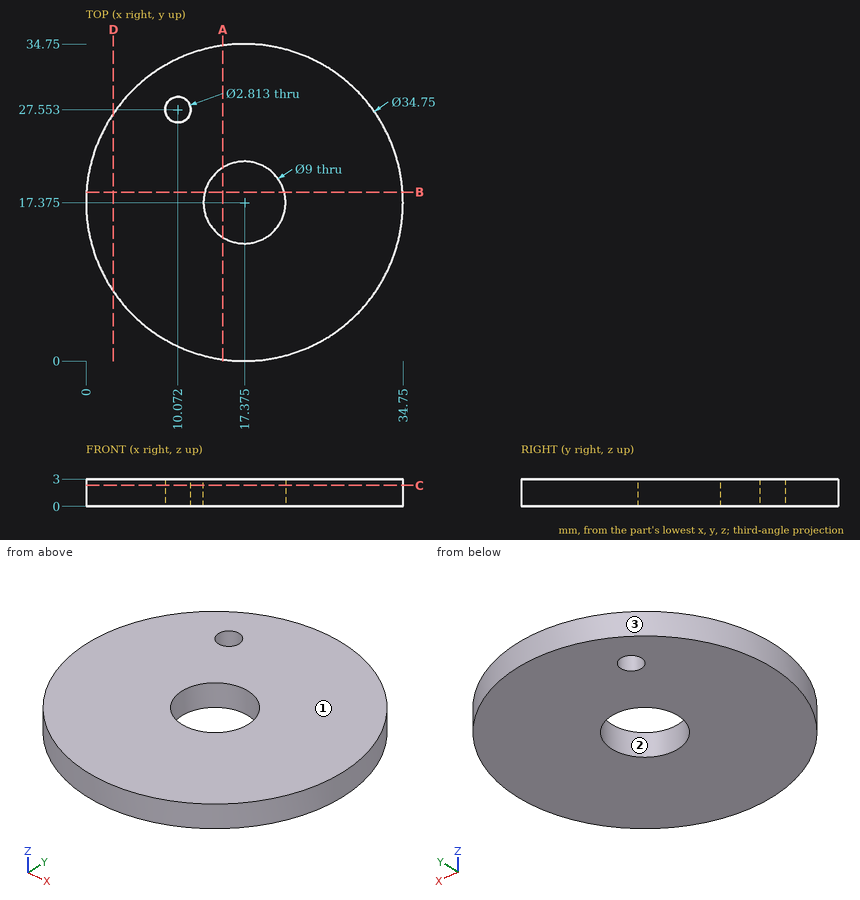
Input: dimensioned drawing with shaded views. Units: mm. Origin: part minimum x, y, z. Coordinates: 2 decimals unless noted, no trailing zeros. Order: outer loops, then holes, each group sorted by start corner. A loop starts at its lowest first (then second) coordinate and runs counter-clockwise, first axis right, second up. Notation, with made-up numbers: M 60,-1.5 L 80,-1.5 A23 cw 80,31.5 Z; hole C 88,85 d11. An arc over 180 degrees is marked long. Answer as CSV lines item,"result".
Q1. Section C-C on z = 2.3. Count the separate pieces of the cut face and the enclosed holes in it.
Answers:
separate pieces,"1"
enclosed holes,"2"
Q2. Section A-A on x = 15. Return the cut outline in (y, z).
Answers:
outline,"M 0.16,0 L 13.55,0 L 13.55,3 L 0.16,3 Z; M 21.2,0 L 34.59,0 L 34.59,3 L 21.2,3 Z"
Q3. Section B-B on y = 18.5. Return the cut outline in (x, z).
Answers:
outline,"M 0.04,0 L 13.02,0 L 13.02,3 L 0.04,3 Z; M 21.73,0 L 34.71,0 L 34.71,3 L 21.73,3 Z"
Q4. Draft query along X for the marked faces 1, 2 and 3. Return one class per face: pulls with the +X half, pulls with the -X half, needs draft (parallel to the pull), parting line crosses it, or undercut.
Answers:
face 1,"needs draft"
face 2,"undercut"
face 3,"parting line crosses it"
Q5. First-contact query: P1, Ø1, axis at x = 25.5, z = 1, coming from the -Y side; P2, Ø1, axis at y = 25, z = 2, coming from the +X side. Flat tips, straight axial feed; report the tip coordinate or a pass-through.
Answers:
P1,"stops at y = 1.76"
P2,"stops at x = 33.22"
Q6. Line query: probe 1 along Y at (x, z) = (9.5, 2.2); probe 2 along Y at (x, z) = (20.5, 1.85) (1 decimal); probe 3 along X at (y, z) = (10, 1.55). Output: solid intervals per line, ascending. Write a range as [from, to].
Answers:
probe 1,"y = [1.89, 26.27], [28.84, 32.86]"
probe 2,"y = [0.3, 14.1], [20.6, 34.5]"
probe 3,"x = [1.64, 33.11]"
Q7. Section D-D on x = 3. Return the cut outline in (y, z) (1 decimal).
Answers:
outline,"M 7.6,0 L 27.1,0 L 27.1,3 L 7.6,3 Z"
